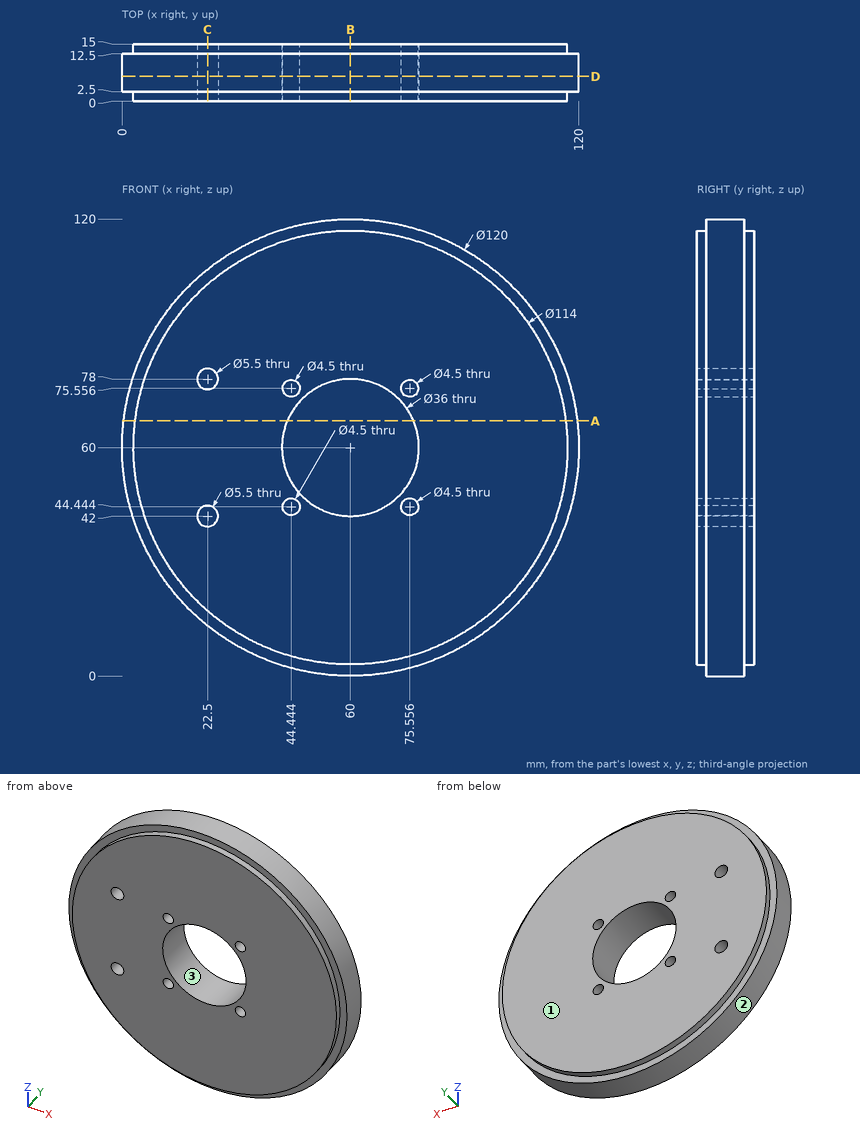
Study the drawing (mm; zero at the part's minimum x, y, z) and answer. Coordinates: 2 decimals unless noted, no trailing zeros. Loops run counter-clockwise (first coordinate to the right, second up) from the corner with the lowest first, then second, coordinate; pieces in that order, holes last. Notation, with made-up numbers: M 10.25,78.25 L 60.25,78.25 A11 ccw 60.25,94.25 Z; hole C 85.25,-2.75 d2. An arc over 180 degrees is marked long. Answer in a Markdown table with one row per item.
1) Find the intervals of material crossed by probe 1 along X at (y, z) = (10.75, 59.5); probe 2 along X at (y, z) = (7, 76.5) (1 decimal); probe 3 along Z at (x, y) = (22.5, 9), in increasing order.
Answers below:
| item | result |
|---|---|
| probe 1 | 0 to 42.01, 77.99 to 120 |
| probe 2 | 2.3 to 20.2, 24.8 to 42.4, 46.5 to 52.8, 67.2 to 73.5, 77.6 to 117.7 |
| probe 3 | 13.16 to 39.25, 44.75 to 75.25, 80.75 to 106.84 |
2) Given pin 1 (4 mm diameter, centred on x = 44.44, z = 44.44, fed in from -Y); pin 2 (2 mm diameter, centred on x = 59.5, y = 7.5, fed in from +Z); pin 3 (8 mm diameter, centred on x = 35, y = 6, fed in from -Z) (1 decimal); pin 4 (4 mm diameter, centred on x = 22.5, y = 2, fed in from -Z) (1 decimal), each flat-ended and moving along its own axis, determine where each tip first touches the part or whether it passes through.
Answers below:
| item | result |
|---|---|
| pin 1 | through |
| pin 2 | z = 120 |
| pin 3 | z = 3.8 |
| pin 4 | z = 11.7 |
3) Find section A-A (z = 67). Determine the outline of the cut face in (x, y), then the cut area to 3 significant figures.
Answers below:
| item | result |
|---|---|
| outline | M 0.41,2.5 L 3.43,2.5 L 3.43,0 L 43.42,0 L 43.42,15 L 3.43,15 L 3.43,12.5 L 0.41,12.5 Z; M 76.58,0 L 116.57,0 L 116.57,2.5 L 119.59,2.5 L 119.59,12.5 L 116.57,12.5 L 116.57,15 L 76.58,15 Z |
| area | 1,260 mm^2 |
4) Find section C-C (x = 22.5). Determine the outline of the cut face in (y, z), then the cut area to 3 significant figures.
Answers below:
| item | result |
|---|---|
| outline | M 0,17.07 L 2.5,17.07 L 2.5,13.16 L 12.5,13.16 L 12.5,17.07 L 15,17.07 L 15,39.25 L 0,39.25 Z; M 0,44.75 L 15,44.75 L 15,75.25 L 0,75.25 Z; M 0,80.75 L 15,80.75 L 15,102.93 L 12.5,102.93 L 12.5,106.84 L 2.5,106.84 L 2.5,102.93 L 0,102.93 Z |
| area | 1,200 mm^2 |
5) Find section B-B (x = 60). Determine the outline of the cut face in (y, z), then the cut area to 3 significant figures.
Answers below:
| item | result |
|---|---|
| outline | M 0,3 L 2.5,3 L 2.5,0 L 12.5,0 L 12.5,3 L 15,3 L 15,42 L 0,42 Z; M 0,78 L 15,78 L 15,117 L 12.5,117 L 12.5,120 L 2.5,120 L 2.5,117 L 0,117 Z |
| area | 1,230 mm^2 |
6) Find section D-D (y = 6.5). Determine the outline of the cut face in (x, z).
Answers below:
| item | result |
|---|---|
| outline | C 60,60 d120; hole C 22.5,42 d5.5; hole C 22.5,78 d5.5; hole C 60,60 d36; hole C 44.44,44.44 d4.5; hole C 44.44,75.56 d4.5; hole C 75.56,44.44 d4.5; hole C 75.56,75.56 d4.5 |
7) Determine the mould class of the marked faces 1, 2 and 3 for opening direction X: released by +X, released by -X, zero draft, split by the parting line, or undercut.
Answers below:
| item | result |
|---|---|
| face 1 | zero draft |
| face 2 | split by the parting line |
| face 3 | undercut |
